The drawing under review shows one solid part. Ordinate dimensions are in mm from its lowest x, y, z. A direction names the side the tool comes from. Give positions to 0.01 mm unless a question says otherwise; leave off trailing zeros. Loops run counter-clockwise (first coordinate to the right, second up) from the corner with the lowest first, then second, coordinate; pieces in that order, holes last. Notation, with made-up numbers: M 25.25,-16 L 82.25,-16 A21 cw 82.25,-8 Z; hole C 69.5,68 d6. An arc over 180 degrees is marked long. Write item = value, one per line. Start each with the question number.
1. We need section B-B on z = 1.4. Give the boundary of the cut face in (x, y), then the cut area to 4 significant figures.
2. We need section C-C on x = 20. Give the boundary of the cut face in (y, z).
3. For the marked faces 1 and 2, list the 3-axis set-ups (+Z, -Z, +X, -X, +Y, -Y) from which the entire face can be reached by the end or side of a thin tool; tool diameter is ignored.
4. For pin 1 (2.5 mm diameter, centred on x = 15, z = 1.5, fed in from +Y); pin 2 (1 mm diameter, centred on y = 8, z = 3, fed in from -X); pin 3 (2.5 mm diameter, centred on y = 19, z = 3.5, fed in from +X), all flat-tipped, find the tip position at first contact; note any pin that passes through.
5. Draft analysis for pull direction X (two halves, no side actions). For the marked faces 3 and 4, state which applies: pulls with the +X half, pulls with the -X half, needs draft (parallel to the pull), parting line crosses it, or undercut.
6. Wall thickness on line 1 along X through (y, z) = (32, 0.9); line 2 along Y through (x, z) = (62.5, 3.85): over which ranges is each line inside the solid? List them lowest first. Write a range as from..to.
7. We need section A-A on y = 15.5. Give the boundary of the cut face in (x, z).
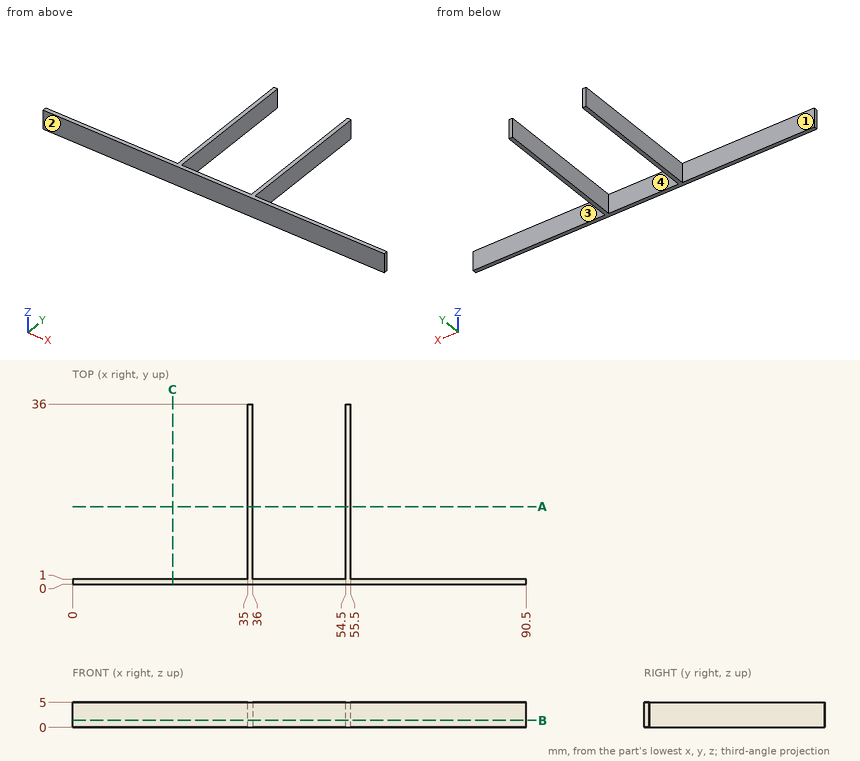
Final values:
q1.outline = M 0,0 L 90.5,0 L 90.5,1 L 55.5,1 L 55.5,36 L 54.5,36 L 54.5,1 L 36,1 L 36,36 L 35,36 L 35,1 L 0,1 Z
q1.area = 160.5 mm²
q2.outline = M 0,0 L 1,0 L 1,5 L 0,5 Z
q3.face_1 = +Z, -Z, -X, +Y
q3.face_2 = +Z, -Z, +X, -X, -Y
q4.pin_1 = 1
q4.pin_2 = 35
q4.pin_3 = 55.5
q5.face_3 = needs draft
q5.face_4 = undercut
q6.line_1 = 35..36, 54.5..55.5
q6.line_2 = 0..1
q7.outline = M 35,0 L 36,0 L 36,5 L 35,5 Z; M 54.5,0 L 55.5,0 L 55.5,5 L 54.5,5 Z
